Geometry check sheet. Reference: drawing and pictorial views, mm from the part's lowest x, y, z. A direction names the side the tool comes from. Coordinates: 2 decimals unless noted, no trailing zeros. Loops run counter-clockwise (first coordinate to the right, second up) from the corner with the lowest first, then second, coordinate; pieces in that order, holes last. Notation, with made-up numbers: (71, -22) - (111, -22) arc R19 cw to (111, 2) - close; hole circle Ø9 at (35.5, 55.25). An arc over 180 degrees is marked (long way). Use a Markdown table: item, result. Add a question column.
1) Draft check along Z on the marked faces 3, 4, 5 and 6. Enter one of: pulls with the +Z half, pulls with the -Z half, needs draft (parallel to the pull), parting line crosses it, or undercut.
2) Sectioned sample at A-A, the plane y = 5. Enter the section's corners in (x, z) (3 decimals), then the cut area to 3 significant figures.
3) Go/stop test with flat-tipped pins: P1, Ø1.6, axis at x = 2.4, y = 5, coming from the -Z side; P2, Ø3, axis at y = 5, z = 5.5, coming from the -X side. Record where each tip stops, or that it passes through.
4) Sectioned sample at B-B, the plane z = 5.5. Enter the section's corners in (x, y) (3 decimals), then the cut area to 3 significant figures.
5) Sectioned sample at D-D, the plane z = 11.25. Enter the section's corners in (x, y).
6) Tool access check on the marked faces 1 and 2. Record the directions out of +Z, -Z, +X, -X, +Y, -Y that give a thin tool (end or side, any length) a straight path to the whole face; none if there is none.
7) Sectioned sample at C-C, the plane x = 2.4. Enter the section's corners in (y, z), then the cut area to 3 significant figures.
8) Thickness scan on line 1 (Y direction, x = 2.4, z = 5.5); line 2 (X direction, y = 5, z = 10.95); line 3 (Y direction, x = 2.4, z = 9.05). Record the ranges inside material, lowest first.
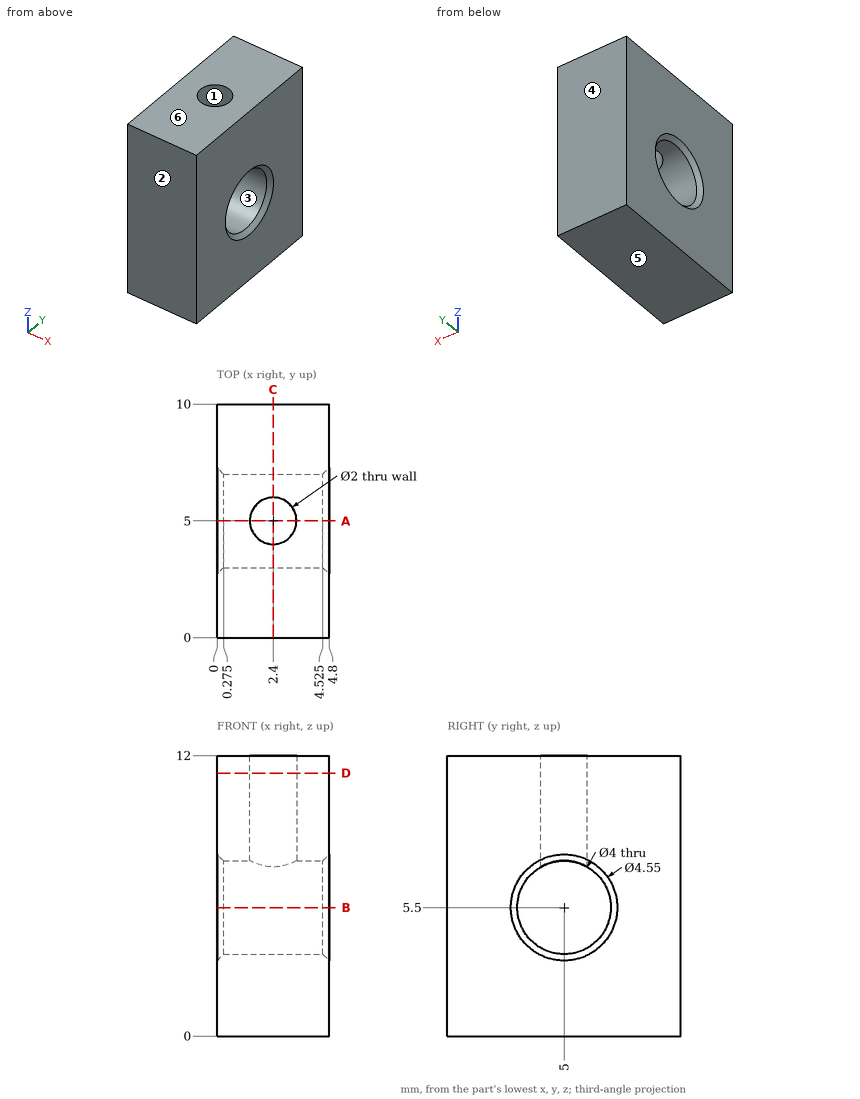
Solved:
| question | item | result |
|---|---|---|
| 1 | face 3 | undercut |
| 1 | face 4 | needs draft |
| 1 | face 5 | pulls with the -Z half |
| 1 | face 6 | pulls with the +Z half |
| 2 | outline | (0, 0) - (4.8, 0) - (4.8, 3.225) - (4.525, 3.5) - (0.275, 3.5) - (0, 3.225) - close; (0, 7.775) - (0.275, 7.5) - (1.4, 7.5) - (1.4, 12) - (0, 12) - close; (3.4, 7.5) - (4.525, 7.5) - (4.8, 7.775) - (4.8, 12) - (3.4, 12) - close |
| 2 | area | 29.2 mm2 |
| 3 | P1 | stops at z = 0 |
| 3 | P2 | passes through |
| 4 | outline | (0, 0) - (4.8, 0) - (4.8, 2.725) - (4.525, 3) - (0.275, 3) - (0, 2.725) - close; (0, 7.275) - (0.275, 7) - (4.525, 7) - (4.8, 7.275) - (4.8, 10) - (0, 10) - close |
| 4 | area | 28.6 mm2 |
| 5 | outline | (0, 0) - (4.8, 0) - (4.8, 10) - (0, 10) - close; hole circle Ø2 at (2.4, 5) |
| 6 | face 1 | +Z |
| 6 | face 2 | +Z, -Z, +X, -X, -Y |
| 7 | outline | (0, 0) - (10, 0) - (10, 12) - (6, 12) - (6, 7.23) arc R2 cw (long way) to (4, 7.23) - (4, 12) - (0, 12) - close |
| 7 | area | 98.3 mm2 |
| 8 | line 1 | y = 0 to 3, 7 to 10 |
| 8 | line 2 | x = 0 to 1.4, 3.4 to 4.8 |
| 8 | line 3 | y = 0 to 4, 6 to 10 |
